Input: dimensioned drawing with shaded views. Units: mm. Origin: part minimum x, y, z. Give positions to 0.01 mm unless a question says otherwise; leave off trailing zeros. Loops run counter-clockwise (first coordinate to the right, second up) from the corner with the lowest first, then second, coordinate; pieces in that order, holes last. Notation, with made-up numbers: (-35, 46.5) -> (-16, 46.5) arc R32 cw to (-16, 81.5) -> close; hole circle Ø11 at (31.25, 88). An arc over 180 degrees is marked (long way). Answer in a Markdown table with one row per item. Add a question column.
1) Section query B-B (y = 95). Return the cut outline in (x, z), plus the area to 3 significant figures.
2) First-contact query: P1, Ø5, axis at x = 198, y = 19.5, coming from the -Z side; P2, Ø6.5, axis at y = 102, z = 4.5, coming from the -X side. Flat tips, straight axial feed; report the tip coordinate or a pass-through.
3) Line query: line 1 (X direction, y = 11, z = 3.5); line 2 (Y direction, x = 21, z = 5.5) (3 decimals). Output: solid intervals per line, ascending. Write a range as from..to.
4) Section query A-A (z = 10). Return the cut outline in (x, y) (3 decimals).
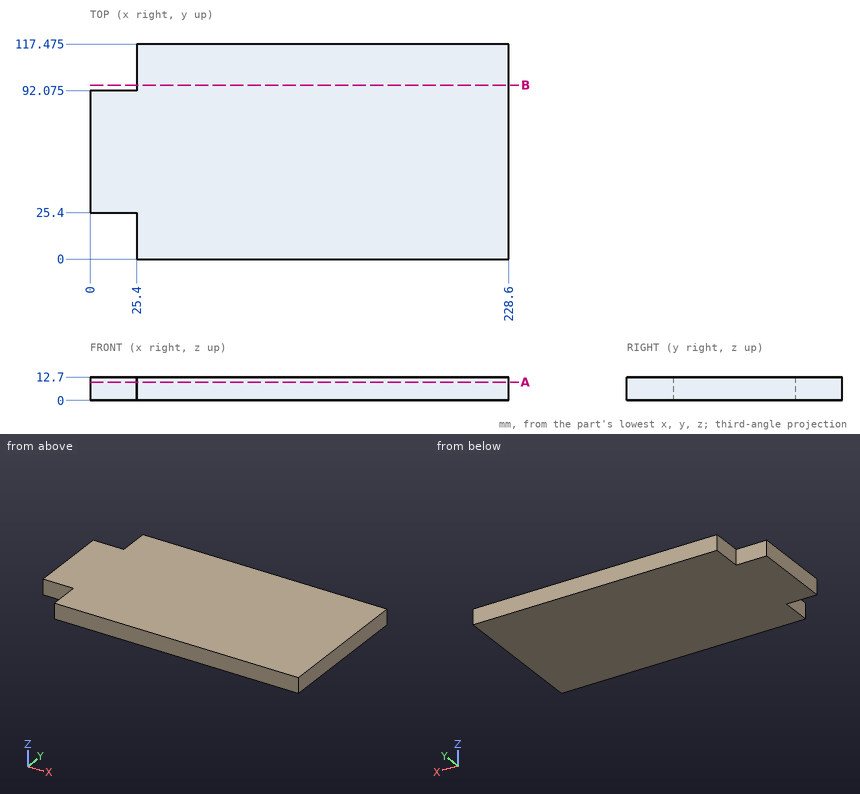
Evaluation:
| question | item | result |
|---|---|---|
| 1 | outline | (25.4, 0) -> (228.6, 0) -> (228.6, 12.7) -> (25.4, 12.7) -> close |
| 1 | area | 2,580 mm² |
| 2 | P1 | z = 0 |
| 2 | P2 | x = 25.4 |
| 3 | line 1 | 25.4..228.6 |
| 3 | line 2 | 25.4..92.075 |
| 4 | outline | (0, 25.4) -> (25.4, 25.4) -> (25.4, 0) -> (228.6, 0) -> (228.6, 117.475) -> (25.4, 117.475) -> (25.4, 92.075) -> (0, 92.075) -> close |
